Verification items for the finished model (mm, model axes). A direction names the side the tool comes from. Round coordinates to 2 decimals unless told otherwise and drop trailing zeros. Order: outer loops, then holes, each group sorted by start corner. A loop starts at its lowest first (then second) coordinate and runs counter-clockwise, first axis right, second up. Notation, with made-up numbers: M 68,40.25 L 110,40.25 A24 cw 110,75.25 Z; hole C 58.5,-17 d6. An arc over 180 degrees is marked long. Return JSON: item names as keys, results as strings. Group by question number.
from build123d import *

# Parameters (mm, degrees)
BOSS_EXTRUDE1_DEPTH = 5
CUT_EXTRUDE1_DEPTH  = 95.158544522
CUT_EXTRUDE2_DEPTH  = 5
SKETCH5_R           = 1.35
BOSS_EXTRUDE2_DEPTH = 10
SKETCH6_R           = 1.7
CUT_EXTRUDE3_DEPTH  = 5


with BuildPart() as part:
    # Sketch1 → Boss-Extrude1 (new body)
    with BuildSketch(Plane.XY):
        Polygon((-30.995, 36.381727213), (-14, 67.5), (14, 67.5), (30.995, 36.381727213), (14.995, 8.668914292), (15, 8.660254038), (15.005, 8.651593784), (47.005, 8.651593784), (65.456714755, -21.625644347), (51.456714755, -45.874355653), (16.01, -45.033320997), (0.01, -17.320508076), (0, -17.320508076), (-0.01, -17.320508076), (-16.01, -45.033320997), (-51.456714755, -45.874355653), (-65.456714755, -21.625644347), (-47.005, 8.651593784), (-15.005, 8.651593784), (-15, 8.660254038), (-14.995, 8.668914292), align=None)
    extrude(amount=BOSS_EXTRUDE1_DEPTH)

    # Sketch2 → Cut-Extrude1 (cut, through all)
    with BuildSketch(Plane.XY.offset(5)):
        Polygon((-28.872149716, 2.651593784), (-12.118974925, -26.293867874), (-19.521225678, -39.114942267), (-48.040387098, -39.791608731), (-58.480737567, -21.708391269), (-43.63514651, 2.651593784), align=None)
        Polygon((-24.113920832, 36.463348484), (-16.71167008, 23.64227409), (16.732422435, 23.678218224), (24.113920832, 36.463348484), (10.440350469, 61.5), (-10.440350469, 61.5), align=None)
        Polygon((43.63514651, 2.651593784), (28.830645005, 2.651593784), (12.139727281, -26.329812008), (19.521225678, -39.114942267), (48.040387098, -39.791608731), (58.480737567, -21.708391269), align=None)
    extrude(amount=-CUT_EXTRUDE1_DEPTH, mode=Mode.SUBTRACT)

    # Sketch3 → Cut-Extrude2 (cut)
    with BuildSketch(Plane(origin=(0, 0, 0), x_dir=(-1, 0, 0), z_dir=(0, 0, -1))):
        with BuildLine():
            Line((6.01040764, 8.131727984), (2.496902196, 4.618222539))
            ThreePointArc((2.496902196, 4.618222539), (-3.712310601, 3.712310601), (-4.618222539, -2.496902196))
            Line((-4.618222539, -2.496902196), (-8.131727984, -6.01040764))
            ThreePointArc((-8.131727984, -6.01040764), (-8.131727984, -8.131727984), (-6.01040764, -8.131727984))
            Line((-6.01040764, -8.131727984), (-2.496902196, -4.618222539))
            ThreePointArc((-2.496902196, -4.618222539), (3.712310601, -3.712310601), (4.618222539, 2.496902196))
            Line((4.618222539, 2.496902196), (8.131727984, 6.01040764))
            ThreePointArc((8.131727984, 6.01040764), (8.131727984, 8.131727984), (6.01040764, 8.131727984))
        make_face()
    extrude(amount=-CUT_EXTRUDE2_DEPTH, mode=Mode.SUBTRACT)

    # Sketch5 → Boss-Extrude2 (add)
    with BuildSketch(Plane.XY.offset(5)):
        with Locations((-45.443044798, 5.870544436)):
            Circle(SKETCH5_R)
        with Locations((-62.08538883, -21.665632507)):
            Circle(SKETCH5_R)
        with Locations((-49.805684066, -42.93470506)):
            Circle(SKETCH5_R)
        with Locations((-17.637483295, -42.290100822)):
            Circle(SKETCH5_R)
        with Locations((27.80556106, 36.419560852)):
            Circle(SKETCH5_R)
        with Locations((12.279704321, 64.600342034)):
            Circle(SKETCH5_R)
        with Locations((-12.279705207, 64.600342034)):
            Circle(SKETCH5_R)
        with Locations((-27.805561947, 36.419560852)):
            Circle(SKETCH5_R)
        with Locations((17.637482409, -42.290100822)):
            Circle(SKETCH5_R)
        with Locations((49.80568318, -42.93470506)):
            Circle(SKETCH5_R)
        with Locations((62.085387944, -21.665632507)):
            Circle(SKETCH5_R)
        with Locations((45.443043912, 5.870544436)):
            Circle(SKETCH5_R)
    extrude(amount=BOSS_EXTRUDE2_DEPTH)

    # Sketch6 → Cut-Extrude3 (cut)
    with BuildSketch(Plane(origin=(0, 0, 0), x_dir=(-1, 0, 0), z_dir=(0, 0, -1))):
        with Locations((-8, 0)):
            Circle(SKETCH6_R)
        with Locations((0, -8)):
            Circle(SKETCH6_R)
        with Locations((8, 0)):
            Circle(SKETCH6_R)
        with Locations((0, 8)):
            Circle(SKETCH6_R)
    extrude(amount=-CUT_EXTRUDE3_DEPTH, mode=Mode.SUBTRACT)


solid = part.part
1. Cross-section at A-A (x = 55). Enter the section's corners in (y, z).
2. Access from +Z, -Z, +X, -X, +Y, -Y to the whole of each face (thin tool, end or side, straight path). Record for faces 5 (the face through (-20.61, -11.62, 2.54)), 6 (the face through (50, -43, 15)).
3. Cross-section at C-C (z = 8.5). Give the number of separate pieces and of enclosed holes in the cut face, plus the area to 3 significant figures.
4. Draft check along Y on faces 1 (the face through (-63.08, -20.75, 9.93)), 2 (the face through (62, -22, 15)), 3 (the face through (4.28, -6.4, 2.46)), 4 (the face through (20.6, -11.64, 2.54)). Enter one of: +Y half, -Y half, draft (parallel to the pull), parting line (faces both ways), or undercut.
5. Cross-section at D-D (x = 22). Enter the section's corners in (y, z), plus the area to 3 significant figures.
6. Thickness scan on line 1 along Y through (x, z) = (8, 2.25); line 2 along Y through (x, z) = (0, 1.1); line 3 along Y through (x, z) = (9, 4.5). Record the ranges inside material, lowest first. Write a range as from..to.
7. Cross-section at B-B (y = -13.5). Enter the section's corners in (x, z).
8. Go/stop test with flat-tipped pins: pin 1 (5.5 mm diameter, centred on x = -8, y = 0, fed in from +Z); pin 2 (1.5 mm diameter, centred on x = 34, z = 1.5, fed in from -Y); pin 3 (3 mm diameter, centred on x = 42.5, y = 4, fed in from -Z); pin 4 (2.5 mm diameter, centred on x = -36, z = 2, fed in from +Y). Record where each tip stops, or that it passes through.
Computed:
{
 "1": {"outline": "M -39.74,0 L -27.74,0 L -27.74,5 L -39.74,5 Z; M -16,0 L -4.47,0 L -4.47,5 L -16,5 Z"},
 "2": {"face 5": "+Z, -Z", "face 6": "+Z, +X, -X, +Y, -Y"},
 "3": {"separate pieces": "12", "enclosed holes": "0", "area": "68.7 mm²"},
 "4": {"face 1": "parting line", "face 2": "draft", "face 3": "undercut", "face 4": "undercut"},
 "5": {"outline": "M -45.18,0 L -39.17,0 L -39.17,5 L -45.18,5 Z; M -9.21,0 L 8.65,0 L 8.65,5 L -9.21,5 Z; M 20.8,0 L 32.8,0 L 32.8,5 L 20.8,5 Z; M 40.33,0 L 52.85,0 L 52.85,5 L 40.33,5 Z", "area": "242 mm²"},
 "6": {"line 1": "y = -31.16..-8.25, -5.88..-1.7, 1.7..23.67, 61.5..67.5", "line 2": "y = -17.32..-9.7, -6.3..-5.25, 5.25..6.3, 9.7..23.66, 61.5..67.5", "line 3": "y = -32.89..-1.37, 1.37..23.67, 61.5..67.5"},
 "7": {"outline": "M -60.5,0 L -53.48,0 L -53.48,5 L -60.5,5 Z; M -19.52,0 L 19.53,0 L 19.53,5 L -19.52,5 Z; M 53.48,0 L 60.5,0 L 60.5,5 L 53.48,5 Z"},
 "8": {"pin 1": "stops at z = 5", "pin 2": "stops at y = -45.48", "pin 3": "stops at z = 0", "pin 4": "stops at y = 8.65"}
}
